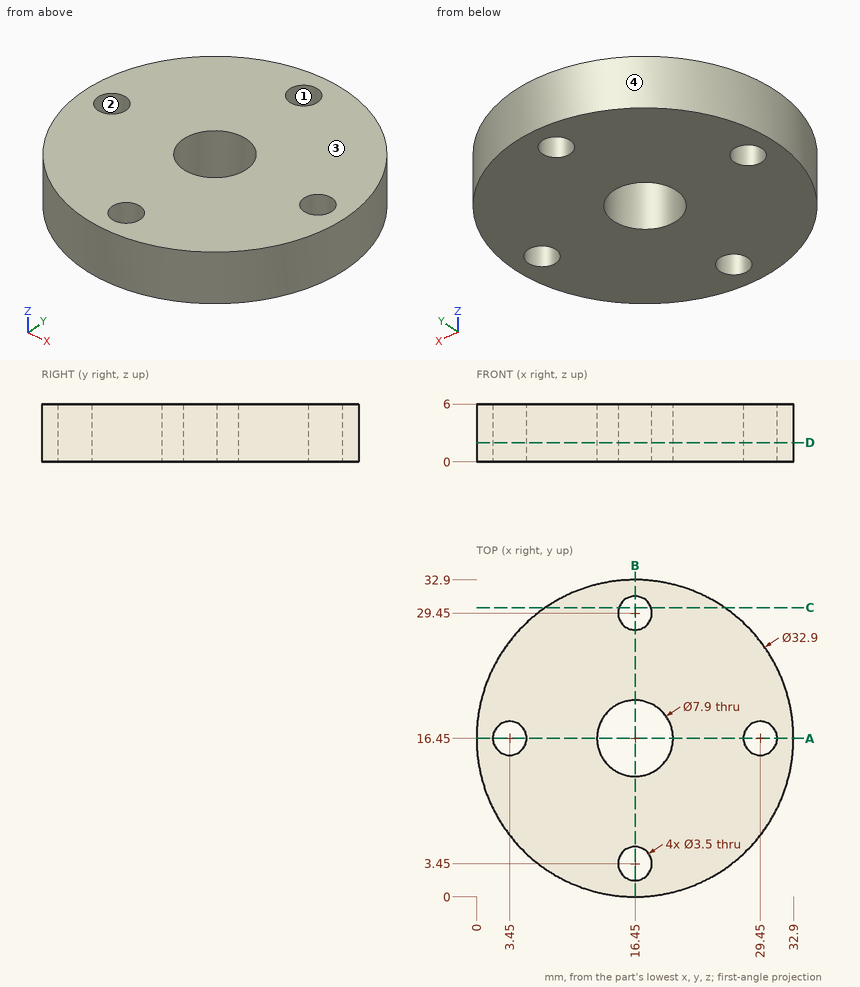
Can you work these out from the drawing? Everything is in mm from the part's minimum corner. Give positions to 0.01 mm unless a question says otherwise; leave off trailing zeros. Loops run counter-clockwise (first coordinate to the right, second up) from the corner with the lowest first, then second, coordinate; pieces in that order, holes last. Notation, with made-up numbers: (58.25, 2) -> (101.25, 2) arc R21 cw to (101.25, 32) -> close; hole circle Ø3 at (31, -29.75). An arc over 180 degrees is marked (long way). Return JSON: item names as keys, results as strings.
Item 1: We'd pull the mould along X, two halves only. Please class the marked faces 1, 2, 3 and 4: +X half, -X half, draft (parallel to the pull), parting line (faces both ways), or undercut.
Geometry results:
{"face 1": "undercut", "face 2": "undercut", "face 3": "draft", "face 4": "parting line"}
Item 2: I need wall thicknesses on L1, parallel to Y at x = 16.45, z = 3; L2, parallel to Y at x = 16, z = 4.6; L3, parallel to Y at x = 2.5, z = 3.55. Which ranges of each line are inside material? Lowest first, please. Write a range as from..to.
Geometry results:
{"L1": "y = 0..1.7, 5.2..12.5, 20.4..27.7, 31.2..32.9", "L2": "y = 0.01..1.76, 5.14..12.53, 20.37..27.76, 31.14..32.89", "L3": "y = 7.73..14.98, 17.92..25.17"}
Item 3: If we section it at A-A on y = 16.45: List the corners of the cut face in (x, z) for me.
Geometry results:
{"outline": "(0, 0) -> (1.7, 0) -> (1.7, 6) -> (0, 6) -> close; (5.2, 0) -> (12.5, 0) -> (12.5, 6) -> (5.2, 6) -> close; (20.4, 0) -> (27.7, 0) -> (27.7, 6) -> (20.4, 6) -> close; (31.2, 0) -> (32.9, 0) -> (32.9, 6) -> (31.2, 6) -> close"}
Item 4: I'm going to push flat-ended pins straight in: pin 1 (3 mm diameter, centred on x = 3.45, y = 16.45, fed in from -Z); pin 2 (1 mm diameter, centred on y = 23, z = 1, fed in from +X); pin 3 (1.5 mm diameter, centred on y = 20, z = 4.5, fed in from -X). Where does each tip first touch, or does it pass through?
Geometry results:
{"pin 1": "passes through", "pin 2": "stops at x = 31.75", "pin 3": "stops at x = 0.24"}
Item 5: If we section it at D-D on z = 2: List the corners of the cut face in (x, y) for me, plus the area to 3 significant figures.
Geometry results:
{"outline": "circle Ø32.9 at (16.45, 16.45); hole circle Ø3.5 at (3.45, 16.45); hole circle Ø7.9 at (16.45, 16.45); hole circle Ø3.5 at (16.45, 3.45); hole circle Ø3.5 at (16.45, 29.45); hole circle Ø3.5 at (29.45, 16.45)", "area": "763 mm²"}
Item 6: If we section it at C-C on y = 30: List the corners of the cut face in (x, z) for me.
Geometry results:
{"outline": "(7.12, 0) -> (14.79, 0) -> (14.79, 6) -> (7.12, 6) -> close; (18.11, 0) -> (25.78, 0) -> (25.78, 6) -> (18.11, 6) -> close"}
